```python
from build123d import *

# Parameters (mm, degrees)
SKETCH1_W           = 56.2
SKETCH1_H           = 100.725
BOSS_EXTRUDE1_DEPTH = 2.38125
SKETCH2_R           = 20.25
SKETCH2_R_2         = 1.5
SKETCH2_R_3         = 3.2639
CUT_EXTRUDE1_DEPTH  = 58.867718224
FILLET1_R           = 2


with BuildPart() as part:
    # Sketch1 → Boss-Extrude1 (new, symmetric)
    with BuildSketch(Plane.XY):
        Rectangle(SKETCH1_W, SKETCH1_H)
    extrude(amount=BOSS_EXTRUDE1_DEPTH, both=True)

    # Sketch2 → Cut-Extrude1 (cut, through all)
    with BuildSketch(Plane.XY.offset(2.38125)):
        with Locations((0, 22.2625)):
            Circle(SKETCH2_R)
        with Locations((-23.5, 45.7625)):
            Circle(SKETCH2_R_2)
        with Locations((23.5, 45.7625)):
            Circle(SKETCH2_R_2)
        with Locations((-23.5, -1.2375)):
            Circle(SKETCH2_R_2)
        with Locations((23.5, -1.2375)):
            Circle(SKETCH2_R_2)
        with Locations((-18.575, -32.9)):
            Circle(SKETCH2_R_3)
        with Locations((18.575, -32.9)):
            Circle(SKETCH2_R_3)
    extrude(amount=-CUT_EXTRUDE1_DEPTH, mode=Mode.SUBTRACT)

    # Fillet1
    fillet1_edges = [part.edges().sort_by_distance(p)[0] for p in [
        (28.1, -50.3625, 0),
        (-28.1, -50.3625, 0),
        (-28.1, 50.3625, 0),
        (28.1, 50.3625, 0),
    ]]
    fillet(fillet1_edges, radius=FILLET1_R)


solid = part.part
```
Verification items for the finished model (mm, model axes). Round coordinates to 2 decimals unless told otherwise and drop trailing zeros. Write each loop counter-clockwise with the first axis right and the second up, starting at its lowest first coordinate (ties: lowest second). Pieces come first, ordered by that corner, then holes. Notation, with made-up numbers: (33, -16) - (74, -16) arc R22 cw to (74, -6) - close; hole circle Ø3 at (2, 75). An arc over 180 degrees is marked (long way). Answer as a JSON object with one key per item and string values. Group by question number.
Q1. Thickness scan on line 1 (Y direction, x = 23.5, z = -2.05); line 2 (X direction, y = 23, z = -1.85); line 3 (X direction, y = -32, z = 1.45). Record the ranges inside material, lowest first.
Q2. Section check C-C, the plane x = 23.5. Enter the section's corners in (y, z), plus the area to 3 significant figures.
Q3. Section check A-A, the plane x = 0. Enter the section's corners in (y, z).
Q4. Section check B-B, the plane y = -32.9. Enter the section's corners in (x, z), plus the area to 3 significant figures.
Q5. Mould release check, pull along X, two halves, no side actions. Record for faces 1 (the flat face through (28.1, -1, 0)), 2 (the flat face through (-28.1, -1, 0)), 3 (the cylindrical face through (22.394, 46.776, 0.033)), 4 (the flat face through (0, -10, -2.381)): released by +X, released by -X, zero draft, split by the parting line, or undercut.
Q6. Section check D-D, the plane y = 5. Enter the section's corners in (x, z), plus the area to 3 significant figures.
Q7. Go/stop test with a flat-tipped pin: pin 1 Ø2.5 at (x, y) = (-23.5, 45.76) entering from -Z. Record where the tip stops, or that it passes through.
Found:
{
 "1": {"line 1": "y = -50.36 to -2.74, 0.26 to 44.26, 47.26 to 50.36", "line 2": "x = -28.1 to -20.24, 20.24 to 28.1", "line 3": "x = -28.1 to -21.71, -15.44 to 15.44, 21.71 to 28.1"},
 "2": {"outline": "(-50.36, -2.38) - (-2.74, -2.38) - (-2.74, 2.38) - (-50.36, 2.38) - close; (0.26, -2.38) - (44.26, -2.38) - (44.26, 2.38) - (0.26, 2.38) - close; (47.26, -2.38) - (50.36, -2.38) - (50.36, 2.38) - (47.26, 2.38) - close", "area": "451 mm^2"},
 "3": {"outline": "(-50.36, -2.38) - (2.01, -2.38) - (2.01, 2.38) - (-50.36, 2.38) - close; (42.51, -2.38) - (50.36, -2.38) - (50.36, 2.38) - (42.51, 2.38) - close"},
 "4": {"outline": "(-28.1, -2.38) - (-21.84, -2.38) - (-21.84, 2.38) - (-28.1, 2.38) - close; (-15.31, -2.38) - (15.31, -2.38) - (15.31, 2.38) - (-15.31, 2.38) - close; (21.84, -2.38) - (28.1, -2.38) - (28.1, 2.38) - (21.84, 2.38) - close", "area": "205 mm^2"},
 "5": {"face 1": "released by +X", "face 2": "released by -X", "face 3": "undercut", "face 4": "zero draft"},
 "6": {"outline": "(-28.1, -2.38) - (-10.59, -2.38) - (-10.59, 2.38) - (-28.1, 2.38) - close; (10.59, -2.38) - (28.1, -2.38) - (28.1, 2.38) - (10.59, 2.38) - close", "area": "167 mm^2"},
 "7": {"pin 1": "passes through"}
}
